Part model, mm, in its own coordinate system. Face numbers are marked on the shaded views. A direction names the side the tool comes from. Round coordinates to 2 decimals unless told otherwise and drop trailing zeros. Loops run counter-clockwise (first coordinate to the right, second up) from the corner with the lowest first, then second, coordinate; pieces in that order, holes last. Notation, with made-up numbers: (-27, 39) -> (14, 39) arc R29 ccw to (14, 69) -> close; hole circle Ø7 at (12, -40). An arc over 180 degrees is marked (long way). Use a Markdown table: item, result. Add a question column.
Item 1: Which spindle directions (+Z, -Z, +X, -X, +Y, -Y) get a long thin tool onto all of the face, cutting with end or side? Do the marked faces 5, 6 and 7. Say none if no direction does.
Item 2: Flat gauge pins, fed straight in: pin 1 (8 mm diameter, centred on x = 58.5, z = -1, fed in from -Y); pin 2 (5.5 mm diameter, centred on x = 8.5, y = 20.5, fed in from +Z); pin 3 (3 mm diameter, centred on x = 54, y = 19.5, fed in from +Z); pin 4 (16 mm diameter, centred on y = 20, z = 0, fed in from -X). Where does each tip first touch, or does it go through?
Item 3: Cut at A-A, the plane x = 47.5. List the corners of the cut face in (y, z).
Item 4: Cut at C-C, the plane x = 62. List the corners of the cut face in (y, z).
Item 5: Cut at B-B, the plane z = 0. List the corners of the cut face in (x, y), plus the area to 3 significant figures.
Item 6: Two-plate mould, pull along Y, no slides. Class the marked faces 1, 2, 3 and 4: pulls with the +Y half, pulls with the -Y half, needs draft (parallel to the pull), parting line crosses it, or undercut.
Item 7: Probe line 1 (Y direction, x = 61.5, z = 0); line 2 (Z direction, x = 49, y = 6); line 3 (Z direction, x = 14, y = 10). List the from-to ranges inside material, lowest first. Write a range as [from, to].
Item 8: Cut at D-D, the plane y = 20. State how many separate pieces and enclosed holes the cut face has, plus the area to 3 significant figures.
```python
from build123d import *

# Parameters (mm, degrees)
SKETCH1_R               = 7.5
BOSS_EXTRUDE1_DEPTH     = 29
CUT_EXTRUDE1_DEPTH      = 65
CUT_EXTRUDE2_DEPTH      = 95.026591983
CUT_EXTRUDE2_DEPTH_BACK = 38
SKETCH4_R               = 7
CUT_EXTRUDE3_DEPTH      = 40
CUT_EXTRUDE6_START      = -12
SKETCH10_R              = 7.5
CUT_EXTRUDE6_DEPTH      = 12
CUT_EXTRUDE7_START      = -4
CUT_EXTRUDE7_DEPTH      = 4


with BuildPart() as part:
    # Sketch1 → Boss-Extrude1 (new, symmetric)
    with BuildSketch(Plane.XY):
        with BuildLine():
            Line((0, 0), (65, 0))
            Line((65, 0), (80, 8.660254038))
            Line((80, 8.660254038), (80, 31.339745962))
            Line((80, 31.339745962), (65, 40))
            Line((65, 40), (36.66060556, 40))
            ThreePointArc((36.66060556, 40), (16.66060556, 35.82575695), (0, 24))
            Line((0, 24), (0, 0))
        make_face()
        with Locations(Location((34, 19, 0), (0, 0, 180))):
            Circle(SKETCH1_R, mode=Mode.SUBTRACT)
    extrude(amount=BOSS_EXTRUDE1_DEPTH, both=True)

    # Sketch2 → Cut-Extrude1 (cut)
    with BuildSketch(Plane(origin=(0, 0, 0), x_dir=(1, 0, 0), z_dir=(0, 1, 0))):
        Polygon((0, 20.995620851), (16, 20.995620851), (16, 15), (54, 15), (54, -15), (16, -15), (16, -21), (0, -21), align=None)
    extrude(amount=CUT_EXTRUDE1_DEPTH, mode=Mode.SUBTRACT)

    # Sketch4 → Cut-Extrude2 (cut, two sides: drawn at the far end of the back side and taken through both)
    with BuildSketch(Plane(origin=(80, 0, 0), x_dir=(0, 0, -1), z_dir=(1, 0, 0)).offset(-CUT_EXTRUDE2_DEPTH_BACK)):
        with Locations(Location((0, 20, 0), (0, 0, 180))):
            Circle(SKETCH4_R)
    extrude(amount=CUT_EXTRUDE2_DEPTH + CUT_EXTRUDE2_DEPTH_BACK, mode=Mode.SUBTRACT)

    # Sketch6 → Cut-Extrude3 (cut)
    with BuildSketch(Plane(origin=(0, 0, 0), x_dir=(1, 0, 0), z_dir=(0, 1, 0))):
        Polygon((65, 29), (80, 29), (80, 14), align=None)
        Polygon((65, -29), (80, -29), (80, -14), align=None)
    extrude(amount=CUT_EXTRUDE3_DEPTH, mode=Mode.SUBTRACT)

    # Sketch10 → Cut-Extrude6 (cut)
    with BuildSketch(Plane.XY.offset(29).offset(CUT_EXTRUDE6_START)):
        with BuildLine():
            Line((18, 34.224221872), (18, 2))
            Line((18, 2), (63, 2))
            Line((63, 2), (63, 38))
            Line((63, 38), (36.66060556, 38))
            ThreePointArc((36.66060556, 38), (27.141221384, 37.046586751), (18, 34.224221872))
        make_face()
        with Locations(Location((34, 19, 0), (0, 0, 180))):
            Circle(SKETCH10_R, mode=Mode.SUBTRACT)
    extrude(amount=CUT_EXTRUDE6_DEPTH, mode=Mode.SUBTRACT)

    # Sketch10_5 → Cut-Extrude7 (cut)
    with BuildSketch(Plane.XY.offset(29).offset(CUT_EXTRUDE7_START)):
        with BuildLine():
            Line((0, 2), (16, 2))
            Line((16, 2), (16, 33.325966555))
            ThreePointArc((16, 33.325966555), (8.226703697, 28.671866064), (1.466424222, 22.64))
            Line((1.466424222, 22.64), (0, 21.058823529))
            Line((0, 21.058823529), (0, 2))
        make_face()
        with BuildLine():
            Line((16, 2), (18, 2))
            Line((18, 2), (18, 34.224221872))
            ThreePointArc((18, 34.224221872), (16.994870724, 33.786514743), (16, 33.325966555))
            Line((16, 33.325966555), (16, 2))
        make_face()
    extrude(amount=CUT_EXTRUDE7_DEPTH, mode=Mode.SUBTRACT)


solid = part.part
```
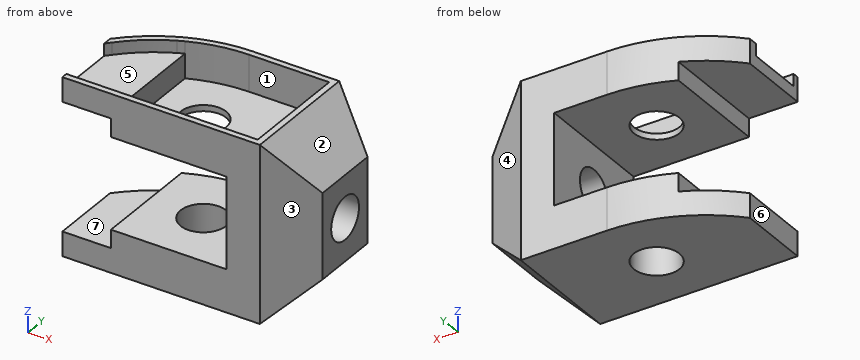
A:
| question | item | result |
|---|---|---|
| 1 | face 5 | +Z |
| 1 | face 6 | +Z, -Z, -X, +Y, -Y |
| 1 | face 7 | -X, +Y, -Y |
| 2 | pin 1 | stops at y = 0 |
| 2 | pin 2 | stops at z = 25 |
| 2 | pin 3 | stops at z = 17 |
| 2 | pin 4 | stops at x = 54 |
| 3 | outline | (0, -29) -> (40, -29) -> (40, -15) -> (0, -15) -> close; (0, 15) -> (40, 15) -> (40, 29) -> (38, 29) -> (38, 17) -> (2, 17) -> (2, 29) -> (0, 29) -> close |
| 4 | outline | (0, -29) -> (40, -29) -> (40, 29) -> (38, 29) -> (38, 17) -> (2, 17) -> (2, 29) -> (0, 29) -> close; hole circle Ø14 at (20, 0) |
| 5 | outline | (54, 0) -> (65, 0) -> (80, 8.66) -> (80, 13) -> (54, 13) -> close; (54, 27) -> (80, 27) -> (80, 31.34) -> (65, 40) -> (54, 40) -> close |
| 5 | area | 546 mm^2 |
| 6 | face 1 | undercut |
| 6 | face 2 | needs draft |
| 6 | face 3 | pulls with the -Y half |
| 6 | face 4 | pulls with the +Y half |
| 7 | line 1 | y = [0, 13], [27, 40] |
| 7 | line 2 | z = [-29, -15], [15, 17] |
| 7 | line 3 | z = [-29, -21], [21, 25] |
| 8 | separate pieces | 4 |
| 8 | enclosed holes | 0 |
| 8 | area | 1,390 mm^2 |
